Geometry check sheet. Reference: the model listing, model coordinates, mm. A direction names the side the tool comes from. Round coordinates to 2 decimals unless told otherwise and drop trailing zeros. Write each loop counter-clockwise with the first axis right and the second up, starting at its lowest first coordinate (ties: lowest second). Pieces come first, ordered by that corner, then holes. Notation, with made-up numbers: M -3.5,80 L 51.5,80 A23 ccw 51.5,117 Z; hole C -6.5,46.25 d4. An arc over 180 degrees is marked long. Use a Markdown table: item, result.
```python
from build123d import *

# Parameters (mm, degrees)
F1_DEPTH  = 64
F4_DEPTH  = 19
F6_DEPTH  = 6
F8_DEPTH  = 6
F9_R      = 19.5
F10_DEPTH = 12
F11_R     = 11.1871907606
F12_DEPTH = 25
F13_W     = 12.5
F13_H     = 70
F14_DEPTH = 25
F16_DEPTH = 70
F17_R     = 7.5
F18_DEPTH = 70
F19_W     = 40
F19_H     = 38.5815599019
F20_DEPTH = 44.501


with BuildPart() as f1:
    # F0 (on Right) → F1 (new body)
    with BuildSketch(Plane.YZ):
        with BuildLine():
            Line((-54.1868201462, -31.8179203436), (85.8131798538, -31.8179203436))
            Line((85.8131798538, -31.8179203436), (85.8131798538, -12.8179203436))
            Line((85.8131798538, -12.8179203436), (-37.4436623397, -12.8179203436))
            ThreePointArc((-37.4436623397, -12.8179203436), (-42.4436623397, -11.4781743814), (-46.1039163775, -7.8179203436))
            Line((-46.1039163775, -7.8179203436), (-71.3920766998, 35.9824581646))
            ThreePointArc((-71.3920766998, 35.9824581646), (-72.6338098814, 42.3791145671), (-69.671246979, 48.1827630296))
            Line((-69.671246979, 48.1827630296), (-49.2803591326, 67.8348507705))
            Line((-49.2803591326, 67.8348507705), (-62.4652653349, 81.5154300139))
            Line((-62.4652653349, 81.5154300139), (-99.1868201462, 46.124365997))
            Line((-99.1868201462, 46.124365997), (-54.1868201462, -31.8179203436))
        make_face()
    extrude(amount=F1_DEPTH)

    # F3 (on face) → F4 (join)
    with BuildSketch(Plane(origin=(0, -70.8105053198, 73.4725537235), x_dir=(1, 0, 0), z_dir=(0, -0.6939424317, 0.7200304865))):
        with BuildLine():
            Line((0, 11.5901203371), (64, 11.5901203371))
            ThreePointArc((64, 11.5901203371), (32, 43.5901203371), (0, 11.5901203371))
        make_face()
    extrude(amount=-F4_DEPTH)

    # F2 (on face) → F6 (cut)
    with BuildSketch(Plane(origin=(0, -54.4176787662, -31.4180614843), x_dir=(1, 0, 0), z_dir=(0, -0.8660254038, -0.5))):
        Polygon((21, 113.3266016841), (21, 89.53828276), (21, 33.53828276), (43, 33.53828276), (43, 89.53828276), (43, 113.3266016841), align=None)
    extrude(amount=-F6_DEPTH, mode=Mode.SUBTRACT)

    # F7 (on face) → F8 (cut)
    with BuildSketch(Plane(origin=(0, -70.8105053198, 73.4725537235), x_dir=(1, 0, 0), z_dir=(0, -0.6939424317, 0.7200304865))):
        with BuildLine():
            Line((21, 41.6400787397), (21, -39.4098796629))
            Line((21, -39.4098796629), (43, -39.4098796629))
            Line((43, -39.4098796629), (43, 41.6400787397))
            ThreePointArc((43, 41.6400787397), (32, 43.5901203371), (21, 41.6400787397))
        make_face()
    extrude(amount=-F8_DEPTH, mode=Mode.SUBTRACT)

    # F9 (on face) → F10 (cut)
    with BuildSketch(Plane(origin=(0, -70.8105053198, 73.4725537235), x_dir=(1, 0, 0), z_dir=(0, -0.6939424317, 0.7200304865))):
        with Locations((32, 11.5901203371)):
            Circle(F9_R)
    extrude(amount=-F10_DEPTH, mode=Mode.SUBTRACT)

    # F11 (on face) → F12 (cut)
    with BuildSketch(Plane(origin=(0, -70.8105053198, 73.4725537235), x_dir=(1, 0, 0), z_dir=(0, -0.6939424317, 0.7200304865))):
        with Locations((32, 11.5901203371)):
            Circle(F11_R)
    extrude(amount=-F12_DEPTH, mode=Mode.SUBTRACT)

    # F13 (on face) → F14 (join)
    with BuildSketch(Plane.XY.offset(-12.8179203436)):
        with Locations((25.75, 35.8131798538)):
            Rectangle(F13_W, F13_H)
        with Locations((38.25, 35.8131798538)):
            Rectangle(F13_W, F13_H)
    extrude(amount=F14_DEPTH)

    # F15 (on face) → F16 (join, through all)
    with BuildSketch(Plane(origin=(0, 70.8131798538, 0), x_dir=(-1, 0, 0), z_dir=(0, 1, 0))):
        with BuildLine():
            Line((-44.5, 12.1820796564), (-19.5, 12.1820796564))
            ThreePointArc((-19.5, 12.1820796564), (-32, 24.6820796564), (-44.5, 12.1820796564))
        make_face()
    extrude(amount=-F16_DEPTH)

    # F17 (on face) → F18 (cut, through all)
    with BuildSketch(Plane(origin=(0, 70.8131798538, 0), x_dir=(-1, 0, 0), z_dir=(0, 1, 0))):
        with Locations((-32, 12.1820796564)):
            Circle(F17_R)
    extrude(amount=-F18_DEPTH, mode=Mode.SUBTRACT)

    # F19 (on face) → F20 (cut, through all)
    with BuildSketch(Plane.YZ.offset(44.5)):
        with Locations((35.8131798538, 13.4728596074)):
            Rectangle(F19_W, F19_H)
    extrude(amount=-F20_DEPTH, mode=Mode.SUBTRACT)


solid = f1.part
```
Item 1: Mould release check, pull along Y, two halves, no side actions. Record for faces 1 (the face through (44.5, 35, -6)), 2 (the face through (31.846, -80.617, 55.688)), 3 (the face through (40.39, -60.18, 67.05)): +Y half, -Y half, draft (parallel to the pull), parting line (faces both ways), or undercut.
Outcome:
| item | result |
|---|---|
| face 1 | draft |
| face 2 | -Y half |
| face 3 | undercut |
Item 2: Cross-section at C-C, the plane y = -44. Count the separate pieces of the cut face and the enclosed holes in it, and give its area (3 significant figures).
Outcome:
| item | result |
|---|---|
| separate pieces | 2 |
| enclosed holes | 1 |
| area | 2,390 mm2 |
Item 3: Cross-section at A-A, the plane y = 33. Record the cut outline in (x, z), and give its area (3 significant figures).
Outcome:
| item | result |
|---|---|
| outline | M 0,-31.82 L 64,-31.82 L 64,-12.82 L 44.5,-12.82 L 44.5,-5.82 L 19.5,-5.82 L 19.5,-12.82 L 0,-12.82 Z |
| area | 1,390 mm2 |
Item 4: Access from +Z, -Z, +X, -X, +Y, -Y to the whole of each face (thin tool, end or side, straight path). Record for faces 4 (the face through (43, -44, 95)), 5 (the face through (33.63, 8.42, 4.86)), 6 (the face through (31.846, -68.625, -0.894)), 7 (the face through (32, 36, -5.818)).
Outcome:
| item | result |
|---|---|
| face 4 | +Z, -Y |
| face 5 | +Y |
| face 6 | -Y |
| face 7 | +Z, +X, -X |
Item 5: Cross-section at B-B, the plane x = 60. Record the cut outline in (y, z).
Outcome:
| item | result |
|---|---|
| outline | M -99.19,46.12 L -54.19,-31.82 L 85.81,-31.82 L 85.81,-12.82 L -37.44,-12.82 A10 cw -46.1,-7.82 L -71.39,35.98 A10 cw -69.67,48.18 L -38.13,78.59 L -51.31,92.27 Z |
Item 6: Go/stop test with flat-tipped pins: pin 1 (6 mm diameter, centred on x = 51.5, y = -32, fed in from +Z); pin 2 (9 mm diameter, centred on x = 32, z = 12.18, fed in from +Y); pin 3 (12.5 mm diameter, centred on y = 53, z = 2.5, fed in from -X). Record where each tip stops, or that it passes through.
Outcome:
| item | result |
|---|---|
| pin 1 | stops at z = 90.83 |
| pin 2 | stops at y = -55.05 |
| pin 3 | stops at x = 19.5 |
Item 7: Material ranges on line 1 along Z through (x, y) = (32, 67); line 2 along Z through (x, y) = (44.5, -49); line 3 along Z through (x, y) = (11.5, -40.5), recorded low to high. Write a range as from..to.
Outcome:
| item | result |
|---|---|
| line 1 | z = -31.82..4.68, 19.68..24.68 |
| line 2 | z = -31.82..-2.8, 68.11..77.83, 89.11..94.49 |
| line 3 | z = -31.82..-12.34, 76.3..94.13 |
